Design review of the part built by this model. Coordinates are the model's own, in mm. A direction names the side the tool comes from. Give positions to 0.01 mm unless a question says otherwise; leave off trailing zeros. Order: outer loops, then holes, each group sorted by start corner. A loop starts at its lowest first (then second) coordinate and runs counter-clockwise, first axis right, second up. Notation, with made-up numbers: (69, 71.25) -> (81, 71.25) arc R30 cw to (81, 97.25) -> close; hole circle Ø6 at (4, 32). An arc over 180 degrees is marked (long way). Return JSON: item names as keys, results as strings.
```python
from build123d import *

# Parameters (mm, degrees)
CUT_EXTRUDE1_REACH = 134.492
SKETCH2_R          = 2.25


with BuildPart() as part:
    # Sketch1 → Revolve1 (revolve)
    with BuildSketch(Plane.XY, mode=Mode.PRIVATE) as revolve1_sk:
        Polygon((17.4, 0), (17.4, 124), (20, 124), (20, 53.11246026), (20.7, 53.11246026), (20.7, 15.85), (23.45, 15.85), (23.45, 10.85), (21.33256308, 10.85), (21.33256308, 7.45), (23.45, 7.45), (23.45, 4), (33, 4), (33, 0), align=None)
    revolve(revolve1_sk.sketch.rotate(Axis((0, 0, 0), (0, 1, 0)), 90), axis=Axis((0, 0, 0), (0, 1, 0)))

    # Sketch2 → Cut-Extrude1 (cut, up to next)
    with BuildSketch(Plane.XZ, mode=Mode.PRIVATE) as cut_extrude1_sk1:
        with Locations(Location((-19.798989873, 19.798989873, 0), (0, 0, 270))):
            Circle(SKETCH2_R)
    cut_extrude1_tool1 = extrude(cut_extrude1_sk1.sketch, amount=-CUT_EXTRUDE1_REACH, mode=Mode.PRIVATE) & part.part
    # Sketch2 → Cut-Extrude1 (cut, up to next)
    with BuildSketch(Plane.XZ, mode=Mode.PRIVATE) as cut_extrude1_sk2:
        with Locations(Location((19.798989873, 19.798989873, 0), (0, 0, 270))):
            Circle(SKETCH2_R)
    cut_extrude1_tool2 = extrude(cut_extrude1_sk2.sketch, amount=-CUT_EXTRUDE1_REACH, mode=Mode.PRIVATE) & part.part
    # Sketch2 → Cut-Extrude1 (cut, up to next)
    with BuildSketch(Plane.XZ, mode=Mode.PRIVATE) as cut_extrude1_sk3:
        with Locations(Location((19.798989873, -19.798989873, 0), (0, 0, 270))):
            Circle(SKETCH2_R)
    cut_extrude1_tool3 = extrude(cut_extrude1_sk3.sketch, amount=-CUT_EXTRUDE1_REACH, mode=Mode.PRIVATE) & part.part
    # Sketch2 → Cut-Extrude1 (cut, up to next)
    with BuildSketch(Plane.XZ, mode=Mode.PRIVATE) as cut_extrude1_sk4:
        with Locations(Location((-19.798989873, -19.798989873, 0), (0, 0, 270))):
            Circle(SKETCH2_R)
    cut_extrude1_tool4 = extrude(cut_extrude1_sk4.sketch, amount=-CUT_EXTRUDE1_REACH, mode=Mode.PRIVATE) & part.part
    add(cut_extrude1_tool1.solids().sort_by_distance((-19.79899, 0, 19.79899))[0], mode=Mode.SUBTRACT)
    add(cut_extrude1_tool2.solids().sort_by_distance((19.79899, 0, 19.79899))[0], mode=Mode.SUBTRACT)
    add(cut_extrude1_tool3.solids().sort_by_distance((19.79899, 0, -19.79899))[0], mode=Mode.SUBTRACT)
    add(cut_extrude1_tool4.solids().sort_by_distance((-19.79899, 0, -19.79899))[0], mode=Mode.SUBTRACT)


solid = part.part
```
Item 1: Mouldability with a two-part tool opening along Y and no side actions: class faces 4 (the face through (21, 10.85, -5)), 5 (the face through (-0.88, 88.06, 19.98)), 6 (the face through (-17, 53.112, -11)) as released by +Y, released by -Y, zero draft, split by the parting line, or undercut.
Result set:
{"face 4": "undercut", "face 5": "zero draft", "face 6": "released by +Y"}
Item 2: Add section A-A (z = 0). Give the boundary of the cut face in (x, y), plus the area to 3 significant figures.
Result set:
{"outline": "(-33, 0) -> (-17.4, 0) -> (-17.4, 124) -> (-20, 124) -> (-20, 53.11) -> (-20.7, 53.11) -> (-20.7, 15.85) -> (-23.45, 15.85) -> (-23.45, 10.85) -> (-21.33, 10.85) -> (-21.33, 7.45) -> (-23.45, 7.45) -> (-23.45, 4) -> (-33, 4) -> close; (17.4, 0) -> (33, 0) -> (33, 4) -> (23.45, 4) -> (23.45, 7.45) -> (21.33, 7.45) -> (21.33, 10.85) -> (23.45, 10.85) -> (23.45, 15.85) -> (20.7, 15.85) -> (20.7, 53.11) -> (20, 53.11) -> (20, 124) -> (17.4, 124) -> close", "area": "868 mm^2"}
Item 3: Add section D-D (y = 70.5). Give the boundary of the cut face in (x, z).
Result set:
{"outline": "circle Ø40 at (0, 0); hole circle Ø34.8 at (0, 0)"}
Item 4: Add section B-B (x = 0). Give the boundary of the cut face in (y, z), plus the area to 3 significant figures.
Result set:
{"outline": "(0, -33) -> (4, -33) -> (4, -23.45) -> (7.45, -23.45) -> (7.45, -21.33) -> (10.85, -21.33) -> (10.85, -23.45) -> (15.85, -23.45) -> (15.85, -20.7) -> (53.11, -20.7) -> (53.11, -20) -> (124, -20) -> (124, -17.4) -> (0, -17.4) -> close; (0, 17.4) -> (124, 17.4) -> (124, 20) -> (53.11, 20) -> (53.11, 20.7) -> (15.85, 20.7) -> (15.85, 23.45) -> (10.85, 23.45) -> (10.85, 21.33) -> (7.45, 21.33) -> (7.45, 23.45) -> (4, 23.45) -> (4, 33) -> (0, 33) -> close", "area": "868 mm^2"}
Item 5: Add section C-C (y = 20). Give the boundary of the cut face in (x, z), plus the area to 3 significant figures.
Result set:
{"outline": "circle Ø41.4 at (0, 0); hole circle Ø34.8 at (0, 0)", "area": "395 mm^2"}
Item 6: Wall thickness on L1, parallel to Y at x = -6, z = -22; L2, parallel to X at y = 51.5, z = -2.5; L3, parallel to Y at x = -26, z = -16.5: over which ranges is each line inside the solid? List them lowest first. Write a range as [from, to].
Result set:
{"L1": "y = [0, 7.45], [10.85, 15.85]", "L2": "x = [-20.55, -17.22], [17.22, 20.55]", "L3": "y = [0, 4]"}
Item 7: Machinability: for faces 1 (the face through (17.602, 1.972, -19.311)), 2 (the face through (-22.5, 4, -7.8)), 3 (the face through (-21.15, 9.13, 2.78)), which of the approach directions +Z, -Z, +X, -X, +Y, -Y give a long, thin tool a straight path to every point of the face, cutting with its end or side? Answer none if there is none.
Result set:
{"face 1": "+Y, -Y", "face 2": "+Y", "face 3": "none"}
Item 8: For pin 1 (6 mm diameter, centred on x = 22.5, y = 14, fed in from -Z); pin 2 (10 mm diameter, centred on y = 101, z = 12.5, fed in from +X); pin 3 (1 mm diameter, centred on x = -11, y = 95.5, fed in from -Z); pin 4 (1.5 mm diameter, centred on x = -22.5, y = 87.5, fed in from +Z), all flat-tipped, find the tip position at first contact; note any pin that passes through.
Result set:
{"pin 1": "stops at z = -13.03", "pin 2": "stops at x = 18.54", "pin 3": "stops at z = -17.02", "pin 4": "passes through"}
